Check sheet for the drawn part. Datum: minimum x, y, z corner. Units: mm. Round coordinates to 2 decimals unless told otherwise and drop trailing zeros. Write each loop counter-clockwise with the first axis right and the second up, starting at its lowest first coordinate (ties: lowest second). Pieces come first, ordered by that corner, then holes. Notation, with made-up numbers: (83.25, -15.75) - (123.25, -15.75) arc R36 ccw to (123.25, 18.25) - close; hole circle Ø7 at (47.25, 41). An arc over 180 degrees is marked (long way). Answer as a JSON object with one key per item and string values. Group by question number.
Item 1: Sectioned sample at D-D on y = 3.7. Record the boundary of the cut face in (x, z), plus the area to 3 significant figures.
Item 2: Gauge pin test, flat ends, axial feed: P1, Ø1.5, axis at x = 35, y = 2.5, coming from the -Z side; P2, Ø2, axis at x = 12, y = 2.5, coming from the +Z side; P3, Ø1.5, axis at y = 4, z = 15.5, coming from the +X side; P4, Ø3, axis at x = 5, z = 19.5, coming from the -Y side. Record the tip position at first contact, or that the pin passes through.
Item 3: Sectioned sample at B-B on z = 24. Record the boundary of the cut face in (x, y).
Item 4: Release check for a two-part mould opening along Z. For the marked faces 1, 2 and 3 record: pulls with the +Z half, pulls with the -Z half, needs draft (parallel to the pull), parting line crosses it, or undercut.
Item 5: Sectioned sample at C-C on z = 37.5. Record the boundary of the cut face in (x, y).
Item 6: Sectioned sample at A-A on x = 24. Record the boundary of the cut face in (y, z).
Item 7: Thickness scan on line 1 (X direction, y = 3.7, z = 24); line 2 (Y direction, x = 23.5, z = 29); line 3 (X direction, y = 0.85, z = 15.5). Record the ranges inside material, lowest first.
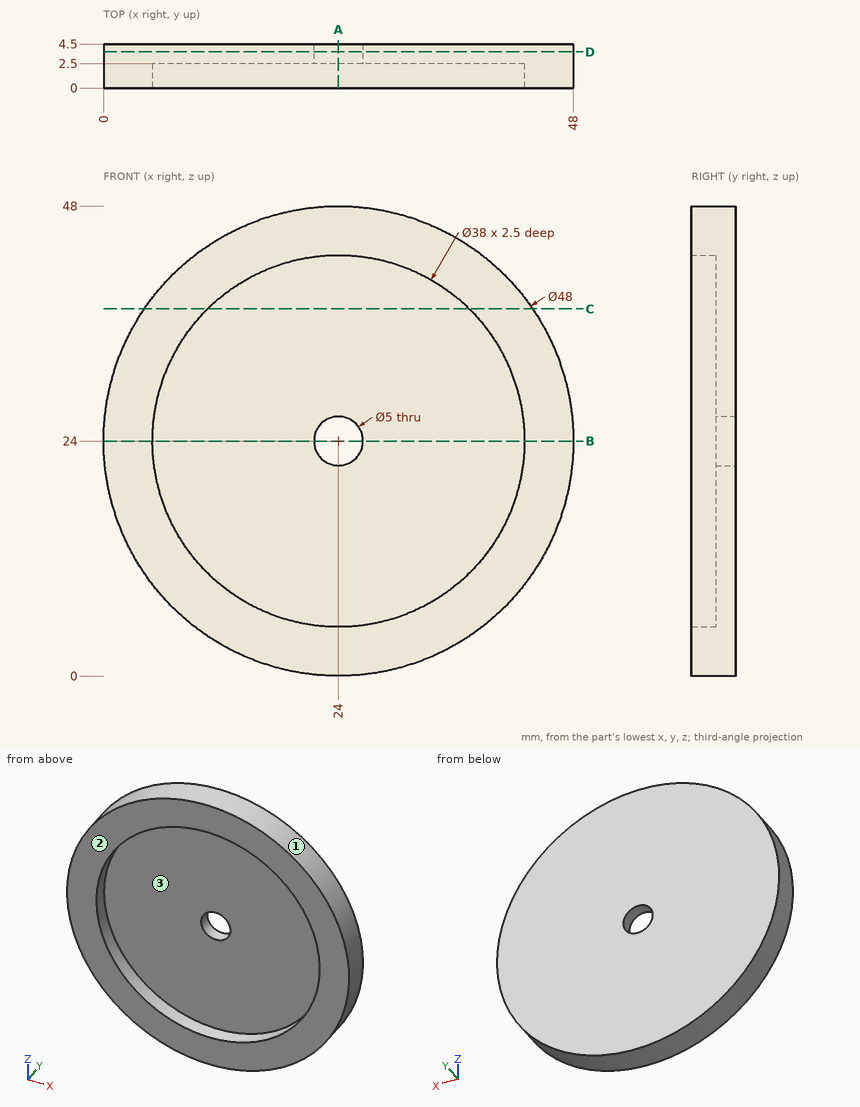
Completed:
{
 "1": {"outline": "circle Ø48 at (24, 24); hole circle Ø5 at (24, 24)", "area": "1,790 mm²"},
 "2": {"P1": "z = 2.3", "P2": "z = 45.33", "P3": "x = 46.71", "P4": "y = 0"},
 "3": {"outline": "(0, 0) - (5, 0) - (5, 2.5) - (21.5, 2.5) - (21.5, 4.5) - (0, 4.5) - close; (26.5, 2.5) - (43, 2.5) - (43, 0) - (48, 0) - (48, 4.5) - (26.5, 4.5) - close"},
 "4": {"face 1": "parting line crosses it", "face 2": "needs draft", "face 3": "undercut"},
 "5": {"outline": "(4.16, 0) - (10.63, 0) - (10.63, 2.5) - (37.37, 2.5) - (37.37, 0) - (43.84, 0) - (43.84, 4.5) - (4.16, 4.5) - close"},
 "6": {"outline": "(0, 0) - (4.5, 0) - (4.5, 21.5) - (2.5, 21.5) - (2.5, 5) - (0, 5) - close; (0, 43) - (2.5, 43) - (2.5, 26.5) - (4.5, 26.5) - (4.5, 48) - (0, 48) - close"},
 "7": {"line 1": "0 to 21.5, 26.5 to 48", "line 2": "2.5 to 4.5", "line 3": "1.56 to 7.01, 40.99 to 46.44"}
}
